Could you check a few things on this drawing? It's one solid part, dimensions in mm from its lowest x, y, z. Round coordinates to 2 decimals unless told otherwise and drop trailing zeros. Loops run counter-clockwise (first coordinate to the right, second up) from the corner with the lowest first, then second, coordinate; pieces in that order, holes last. Notation, with made-up numbers: (61.5, 23.5) -> (97.5, 23.5) arc R10 ccw to (97.5, 37.5) -> close; hole circle Ø6 at (10, 17). An arc over 180 degrees is marked (long way). Write each question's results on one line, items separated by ' | '.
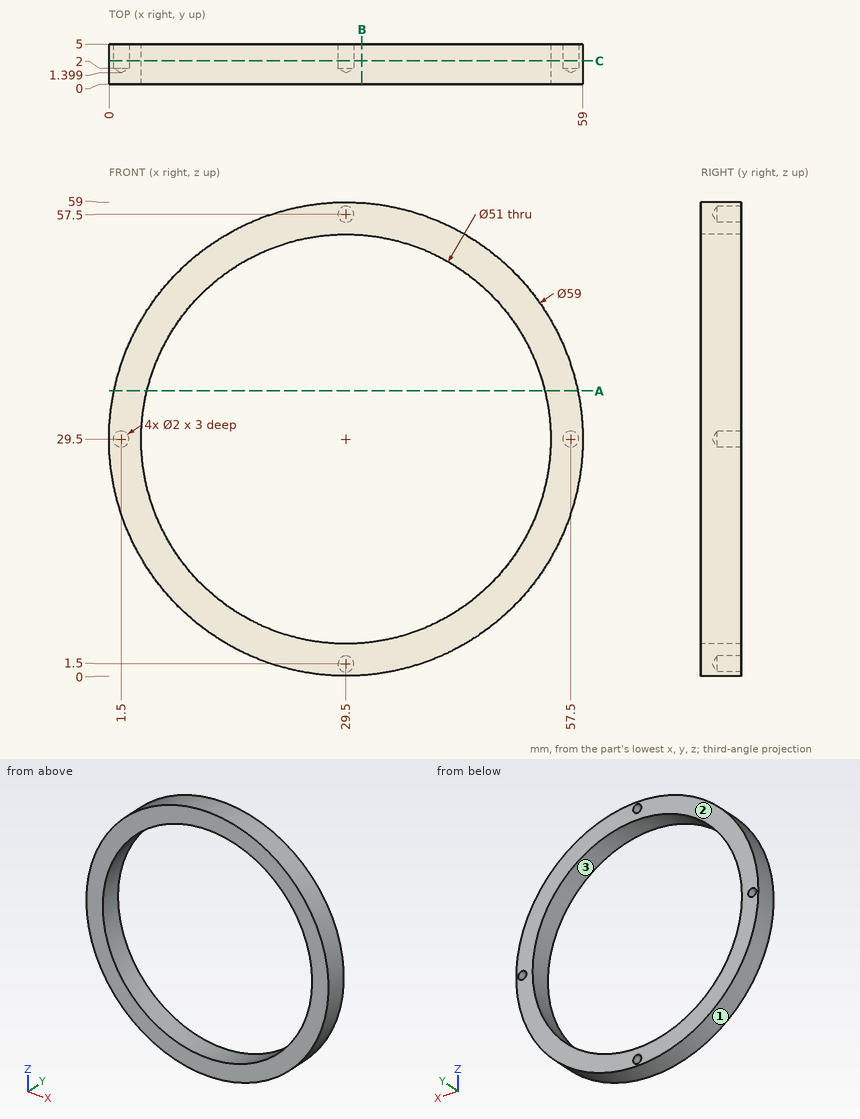
1) I need wall thicknesses on line 1 (Z direction, x = 29.5, y = 2.55); line 2 (Z direction, x = 29.5, y = 1.3); line 3 (X direction, y = 1.1, z = 39.5). Which ranges of each line are inside material? Lowest first, please.
Model answer:
line 1: z = 0 to 0.5, 2.5 to 4, 55 to 56.5, 58.5 to 59 | line 2: z = 0 to 4, 55 to 59 | line 3: x = 1.75 to 6.04, 52.96 to 57.25
2) If we mould it in two halves opening along X, with no side actions, what happens to the marked faces 1, 2 and 3? For each: released by +X, released by -X, zero draft, split by the parting line, or undercut.
Model answer:
face 1: split by the parting line | face 2: zero draft | face 3: undercut
3) I want a section at A-A, the plane z = 35.5. Write out the boundary of the cut face in (x, y).
Model answer:
outline: (0.62, 0) -> (4.72, 0) -> (4.72, 5) -> (0.62, 5) -> close; (54.28, 0) -> (58.38, 0) -> (58.38, 5) -> (54.28, 5) -> close
4) I want a section at C-C, the plane y = 2.9. Write out the boundary of the cut face in (x, z).
Model answer:
outline: circle Ø59 at (29.5, 29.5); hole circle Ø2 at (1.5, 29.5); hole circle Ø51 at (29.5, 29.5); hole circle Ø2 at (29.5, 1.5); hole circle Ø2 at (29.5, 57.5); hole circle Ø2 at (57.5, 29.5)
5) I want a section at B-B, the plane x = 31.5. Write out the boundary of the cut face in (y, z).
Model answer:
outline: (0, 0.07) -> (5, 0.07) -> (5, 4.08) -> (0, 4.08) -> close; (0, 54.92) -> (5, 54.92) -> (5, 58.93) -> (0, 58.93) -> close
6) I'm going to push flat-ended pins straight in: pin 1 (1 mm diameter, centred on x = 19.5, y = 4, fed in from +Z); pin 2 (2 mm diameter, centred on y = 3, z = 22, fed in from -X) (3 decimals); pin 3 (3 mm diameter, centred on y = 1.5, z = 44.5, fed in from -X). Where does each tip first touch, or does it pass through?
Model answer:
pin 1: stops at z = 57.43 | pin 2: stops at x = 0.725 | pin 3: stops at x = 3.27
